Geometry: final body of the model. Coordinates: model frame, mm. A direction names the side the tool comes from. Coordinates: 2 decimals unless noted, no trailing zeros. Order: outer loops, then holes, each group sorted by start corner. A loop starts at its lowest first (then second) coordinate and runs counter-clockwise, first axis right, second up. Notation, with made-up numbers: (71, 34.5) -> (123, 34.5) arc R22 ccw to (123, 52.5) -> close; hole circle Ø1 at (47.5, 73.5). An arc over 180 degrees is marked (long way). Answer in a Markdown table with one row per item. Add a question column.
1) Ray query, line 1 (Y direction, x = 2.5, z = 2.5); line 2 (Y direction, x = 3.75, z = -4.25); line 3 (Y direction, x = -1.25, z = -2). Return the intervals inside material, ascending. Write a range as from..to.
2) Section query D-D on y = -4.5. Return the cut outline in (x, z), then the cut area to 3 significant figures.
3) Section query A-A on z = -4. Return the cut outline in (x, y), then the cut area to 4 significant figures.
4) Pull-direction query (Y, two-part tool) for faces 6 (the face through (0, 13, -7)), 7 (the face through (0.084, 0.371, 13.616)), 8 (the face through (4.028, -13.254, 2.506)); classes: +Y half, -Y half, draft (parallel to the pull), parting line (faces both ways), or undercut.
5) Contact query for flat-ended pins moving along their axis: P1, Ø3, axis at x = -4.5, z = -5.5, coming from the -Y side; P2, Ø4, axis at x = -2, y = -2, coming from the +Z side; P3, Ø1.5, axis at y = -4.5, z = 0, coming from the +X side. Output: stop coordinate, or through.
6) Set-up query: faces 1 (the face through (4, 11, -4)), 2 (the face through (4, -18.8, 2.5)), 3 (the face through (-2, 6, 1)), 4 (the face through (-4, -18.8, 2.5)), 5 (the face through (0, 6, -1)). Return all of +Z, -Z, +X, -X, +Y, -Y with unobstructed straight access to the full face (end or side cutting, diameter ignored); none if empty.
7) Section query B-B on x = 1.5. Return the cut outline in (y, z), then the cut area to 3 significant figures.
8) Section query C-C on z = -0.5. Return the cut outline in (x, y), then the cut area to 3 significant figures.
```python
from build123d import *

# Parameters (mm, degrees)
BOSS_EXTRUDE1_DEPTH     = 6
CHAMFER1_SIZE           = 0.5
CHAMFER2_SIZE           = 0.5
SKETCH3_W               = 4
SKETCH3_H               = 4
BOSS_EXTRUDE2_DEPTH     = 2
CUT_EXTRUDE1_START      = 28.757553028
CUT_EXTRUDE1_DEPTH      = 32.757553028
CHAMFER3_SIZE           = 1
CUT_EXTRUDE2_DEPTH      = 27.277019429
CUT_EXTRUDE2_DEPTH_BACK = 27.277019429
CUT_EXTRUDE3_DEPTH      = 27.277019429
CUT_EXTRUDE3_DEPTH_BACK = 27.277019429


with BuildPart() as part:
    # Sketch1 → Boss-Extrude1 (new, symmetric)
    with BuildSketch(Plane.YZ):
        with BuildLine():
            Line((-21, 0), (-21, -9))
            Line((-21, -9), (-8, -9))
            Line((-8, -9), (-8, 3))
            Line((-8, 3), (8, 3))
            Line((8, 3), (8, -7))
            Line((8, -7), (21, -7))
            Line((21, -7), (21, 0))
            ThreePointArc((21, 0), (0, 13.61916848), (-21, 0))
        make_face()
    extrude(amount=BOSS_EXTRUDE1_DEPTH, both=True)

    # Chamfer1
    chamfer1_edges = [part.edges().sort_by_distance(p)[0] for p in [
        (6, -8, -3),
        (6, 0, 3),
        (6, 8, -2),
    ]]
    chamfer(chamfer1_edges, length=CHAMFER1_SIZE)

    # Chamfer2
    chamfer2_edges = [part.edges().sort_by_distance(p)[0] for p in [
        (-6, -8, -3),
        (-6, 8, -2),
        (-6, 0, 3),
    ]]
    chamfer(chamfer2_edges, length=CHAMFER2_SIZE)

    # Sketch3 → Boss-Extrude2 (add, symmetric)
    with BuildSketch(Plane.YZ):
        with Locations((-6, 1)):
            Rectangle(SKETCH3_W, SKETCH3_H)
    boss_extrude2 = extrude(amount=BOSS_EXTRUDE2_DEPTH, both=True)

    # Mirror1: Boss-Extrude2 across plane
    add(boss_extrude2.mirror(Plane.ZX))

    # Sketch4 → Cut-Extrude1 (cut)
    with BuildSketch(Plane.YZ.offset(6).offset(CUT_EXTRUDE1_START)):
        with BuildLine():
            Line((-11, -9), (-11, -1))
            ThreePointArc((-11, -1), (-13.308790472, 2.534537402), (-17.525839358, 2.334620458))
            ThreePointArc((-17.525839358, 2.334620458), (-18.784311125, 2.485384213), (-18.884110874, 3.748919297))
            ThreePointArc((-18.884110874, 3.748919297), (-20.029956915, 1.924071221), (-21, 0))
            Line((-21, 0), (-21, -9))
            Line((-21, -9), (-11, -9))
        make_face()
        with BuildLine():
            Line((21, -7), (21, 0))
            ThreePointArc((21, 0), (20.029956915, 1.924071221), (18.884110874, 3.748919297))
            ThreePointArc((18.884110874, 3.748919297), (18.784311125, 2.485384213), (17.525839358, 2.334620458))
            ThreePointArc((17.525839358, 2.334620458), (13.308790472, 2.534537402), (11, -1))
            Line((11, -1), (11, -7))
            Line((11, -7), (21, -7))
        make_face()
    cut_extrude1 = extrude(amount=-CUT_EXTRUDE1_DEPTH, mode=Mode.SUBTRACT)

    # Mirror2: Cut-Extrude1 across plane
    add(cut_extrude1.mirror(Plane(origin=(0, 0, 0), x_dir=(0, 0, 1), z_dir=(1, 0, 0))), mode=Mode.SUBTRACT)

    # Chamfer3
    chamfer3_edges = [part.edges().sort_by_distance(p)[0] for p in [
        (0, 21, -7),
    ]]
    chamfer(chamfer3_edges, length=CHAMFER3_SIZE)

    # Sketch5 → Cut-Extrude2 (cut, two sides: drawn at the far end of the back side and taken through both)
    with BuildSketch(Plane.YZ.offset(2).offset(-CUT_EXTRUDE2_DEPTH_BACK)):
        with BuildLine():
            Line((-19, -4.5), (-15, -4.5))
            ThreePointArc((-15, -4.5), (-13.5, -6), (-15, -7.5))
            Line((-15, -7.5), (-19, -7.5))
            ThreePointArc((-19, -7.5), (-20.5, -6), (-19, -4.5))
        make_face()
    extrude(amount=CUT_EXTRUDE2_DEPTH + CUT_EXTRUDE2_DEPTH_BACK, mode=Mode.SUBTRACT)

    # Sketch6 → Cut-Extrude3 (cut, two sides: drawn at the far end of the back side and taken through both)
    with BuildSketch(Plane.YZ.offset(2).offset(-CUT_EXTRUDE3_DEPTH_BACK)):
        with BuildLine():
            Line((19, -5.5), (15, -5.5))
            ThreePointArc((15, -5.5), (13.5, -4), (15, -2.5))
            Line((15, -2.5), (19, -2.5))
            ThreePointArc((19, -2.5), (20.5, -4), (19, -5.5))
        make_face()
    extrude(amount=CUT_EXTRUDE3_DEPTH + CUT_EXTRUDE3_DEPTH_BACK, mode=Mode.SUBTRACT)


solid = part.part
```
Result:
| question | item | result |
|---|---|---|
| 1 | line 1 | -18.8..-17.24, -13.24..-8, 8..13.24, 17.24..18.8 |
| 1 | line 2 | -11..-8, 8..11 |
| 1 | line 3 | -21..-8, 8..21 |
| 2 | outline | (-6, 3.5) -> (-5.5, 3) -> (-2, 3) -> (-2, -1) -> (2, -1) -> (2, 3) -> (5.5, 3) -> (6, 3.5) -> (6, 13.17) -> (-6, 13.17) -> close |
| 2 | area | 138 mm2 |
| 3 | outline | (-6, -11) -> (-2, -11) -> (-2, -21) -> (2, -21) -> (2, -11) -> (6, -11) -> (6, -8.5) -> (5.5, -8) -> (-5.5, -8) -> (-6, -8.5) -> close; (-6, 8.5) -> (-5.5, 8) -> (5.5, 8) -> (6, 8.5) -> (6, 11) -> (2, 11) -> (2, 13.5) -> (-2, 13.5) -> (-2, 11) -> (-6, 11) -> close; (-2, 20.5) -> (2, 20.5) -> (2, 21) -> (-2, 21) -> close |
| 3 | area | 123.5 mm2 |
| 4 | face 6 | draft |
| 4 | face 7 | parting line |
| 4 | face 8 | undercut |
| 5 | P1 | y = -11 |
| 5 | P2 | z = 13.62 |
| 5 | P3 | x = 2 |
| 6 | face 1 | -Z, +X, +Y |
| 6 | face 2 | +X |
| 6 | face 3 | -Z, -X |
| 6 | face 4 | -X |
| 6 | face 5 | -Z, +X, -X |
| 7 | outline | (-21, -9) -> (-8, -9) -> (-8, -1) -> (-4, -1) -> (-4, 3) -> (4, 3) -> (4, -1) -> (8, -1) -> (8, -7) -> (20, -7) -> (21, -6) -> (21, 0) arc R23 ccw to (-21, 0) -> close; hole (-19, -7.5) -> (-15, -7.5) arc R1.5 ccw to (-15, -4.5) -> (-19, -4.5) arc R1.5 ccw to start; hole (15, -5.5) -> (19, -5.5) arc R1.5 ccw to (19, -2.5) -> (15, -2.5) arc R1.5 ccw to start |
| 7 | area | 565 mm2 |
| 8 | outline | (-6, -11.06) -> (-2, -11.06) -> (-2, -21) -> (2, -21) -> (2, -11.06) -> (6, -11.06) -> (6, -8.5) -> (5.5, -8) -> (2, -8) -> (2, -4) -> (-2, -4) -> (-2, -8) -> (-5.5, -8) -> (-6, -8.5) -> close; (-6, 8.5) -> (-5.5, 8) -> (-2, 8) -> (-2, 4) -> (2, 4) -> (2, 8) -> (5.5, 8) -> (6, 8.5) -> (6, 11.06) -> (2, 11.06) -> (2, 21) -> (-2, 21) -> (-2, 11.06) -> (-6, 11.06) -> close |
| 8 | area | 184 mm2 |
